```python
from build123d import *

# Parameters (mm, degrees)
SKETCH_1_W          = 110
SKETCH_1_H          = 66
SKETCH_1_R          = 1.7
EXTRUDE_1_DEPTH     = 4
CUT_EXTRUDE_1_DEPTH = 10
FILLET_1_R          = 4


with BuildPart() as part:
    # 草图1 → 凸台-拉伸1 (new body)
    with BuildSketch(Plane(origin=(0, 0, 0), x_dir=(1, 0, 0), z_dir=(0, 1, 0))):
        with Locations((55, 33)):
            Rectangle(SKETCH_1_W, SKETCH_1_H)
        with Locations(Location((5, 45, 0), (0, 0, 270))):
            Circle(SKETCH_1_R, mode=Mode.SUBTRACT)
        with Locations(Location((5, 5, 0), (0, 0, 270))):
            Circle(SKETCH_1_R, mode=Mode.SUBTRACT)
        with Locations(Location((105, 5, 0), (0, 0, 90))):
            Circle(SKETCH_1_R, mode=Mode.SUBTRACT)
        with Locations(Location((105, 45, 0), (0, 0, 90))):
            Circle(SKETCH_1_R, mode=Mode.SUBTRACT)
        with Locations(Location((15, 63, 0), (0, 0, 270))):
            Circle(SKETCH_1_R, mode=Mode.SUBTRACT)
        with Locations(Location((35, 63, 0), (0, 0, 270))):
            Circle(SKETCH_1_R, mode=Mode.SUBTRACT)
        with Locations(Location((75, 63, 0), (0, 0, 90))):
            Circle(SKETCH_1_R, mode=Mode.SUBTRACT)
        with Locations(Location((95, 63, 0), (0, 0, 90))):
            Circle(SKETCH_1_R, mode=Mode.SUBTRACT)
    extrude(amount=EXTRUDE_1_DEPTH)

    # 草图2 → 切除-拉伸1 (cut)
    with BuildSketch(Plane.XZ):
        Polygon((100, -56), (100, -10), (28.485134293, -56), align=None)
        Polygon((10, -56), (81.514865707, -10), (10, -10), align=None)
    extrude(amount=-CUT_EXTRUDE_1_DEPTH, mode=Mode.SUBTRACT)

    # 圆角1
    fillet_1_edges = [part.edges().sort_by_distance(p)[0] for p in [
        (10, 2, -56),
        (10, 2, -10),
        (81.514865707, 2, -10),
        (100, 2, -56),
        (28.485134293, 2, -56),
        (100, 2, -10),
    ]]
    fillet(fillet_1_edges, radius=FILLET_1_R)


solid = part.part
```
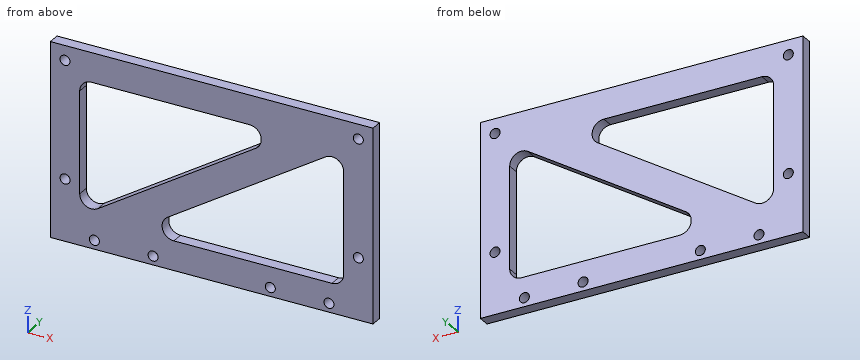
Verification items for the finished model (mm, model axes). Give positions to 0.01 mm unless a question says otherwise; leave off trailing zeros. Loops run counter-clockwise (first coordinate to the right, second up) from the corner with the lowest first, then second, coordinate; pieces in that order, holes last.
1. Section check D-D, the plane x = 24. Enter the section's corners in (y, z).
2. Go/stop test with a flat-tipped pin: pin 1 Ø4 at (x, z) = (5, -5) entering from -Y. Record where the tip stops, or that it passes through.
3. Thickness scan on line 1 (X direction, y = 1.6, z = -5); line 2 (X direction, y = 0.8, z = -63); line 3 (X direction, y = 2.1, z = -44.5). Record the ranges inside material, lowest first.
4. Section check C-C, the plane y = 1.4. Count the separate pieces of the cut face and the enclosed holes in it, then the cut area to 3 significant figures.
5. Section check B-B, the plane z = -63. Enter the section's corners in (x, y), then the cut area to 3 significant figures.
6. Section check A-A, the plane x = 105. Enter the section's corners in (y, z).
Geometry says:
1. outline: (0, -66) - (4, -66) - (4, -46.99) - (0, -46.99) - close; (0, -10) - (4, -10) - (4, 0) - (0, 0) - close
2. pin 1: stops at y = 0
3. line 1: x = 0 to 3.3, 6.7 to 103.3, 106.7 to 110
3. line 2: x = 0 to 13.3, 16.7 to 33.3, 36.7 to 73.3, 76.7 to 93.3, 96.7 to 110
3. line 3: x = 0 to 3.38, 6.62 to 10, 27.88 to 46.36, 100 to 103.38, 106.62 to 110
4. separate pieces: 1
4. enclosed holes: 10
4. area: 4,000 mm2
5. outline: (0, 0) - (13.3, 0) - (13.3, 4) - (0, 4) - close; (16.7, 0) - (33.3, 0) - (33.3, 4) - (16.7, 4) - close; (36.7, 0) - (73.3, 0) - (73.3, 4) - (36.7, 4) - close; (76.7, 0) - (93.3, 0) - (93.3, 4) - (76.7, 4) - close; (96.7, 0) - (110, 0) - (110, 4) - (96.7, 4) - close
5. area: 386 mm2
6. outline: (0, -66) - (4, -66) - (4, -46.7) - (0, -46.7) - close; (0, -43.3) - (4, -43.3) - (4, -6.7) - (0, -6.7) - close; (0, -3.3) - (4, -3.3) - (4, 0) - (0, 0) - close
